Can you work these out from the drawing? Everything is in mm from the part's minimum corner. A direction names the side the tool comes from. Round coordinates to 2 decimals unless told otherwise and drop trailing zeros. Order: outer loops, then holes, each group sorted by start corner. A loop starts at its lowest first (then second) coordinate and runs counter-clockwise, first axis right, second up. Notation, with made-up numbers: M -6.5,14.25 L 36.5,14.25 A15 cw 36.5,40.25 Z; hole C 75,-11 d2. An arc over 180 degrees is marked long. Write each question's results on one line, items separated by ' | '. Start each with the question number.
1. I'm going to push flat-ended pins straight in: pin 1 (1 mm diameter, centred on y = 51.5, z = 5.5, fed in from -X); pin 2 (2 mm diameter, centred on x = 30.5, z = 12.5, fed in from +Y); pin 3 (10 mm diameter, centred on x = 60.5, y = 16, fed in from +Z). Where does each tip first touch, or does it pass through?
2. Suppose I cut it at A-A on x = 10. Write out the boundary of the cut face in (y, z).
3. Suppose I cut it at B-B on y = 68. Write out the boundary of the cut face in (x, z).
4. Suppose I cut it at C-C on z = 9. Write out the boundary of the cut face in (x, y).
5. Please list where these lines run through material, in increasing order: L1, parallel to Z at x = 76, y = 68; L2, parallel to X at y = 34.5, z = 16; L3, parallel to Y at x = 52, z = 14.
6. For the marked faces 1 and 2, which set-ups out of +Z, -Z, +X, -X, +Y, -Y let a thin tool reach every point of the face, with its end or its side?
7. Suppose I cut it at D-D on z = 2.75. Write out the boundary of the cut face in (x, y).
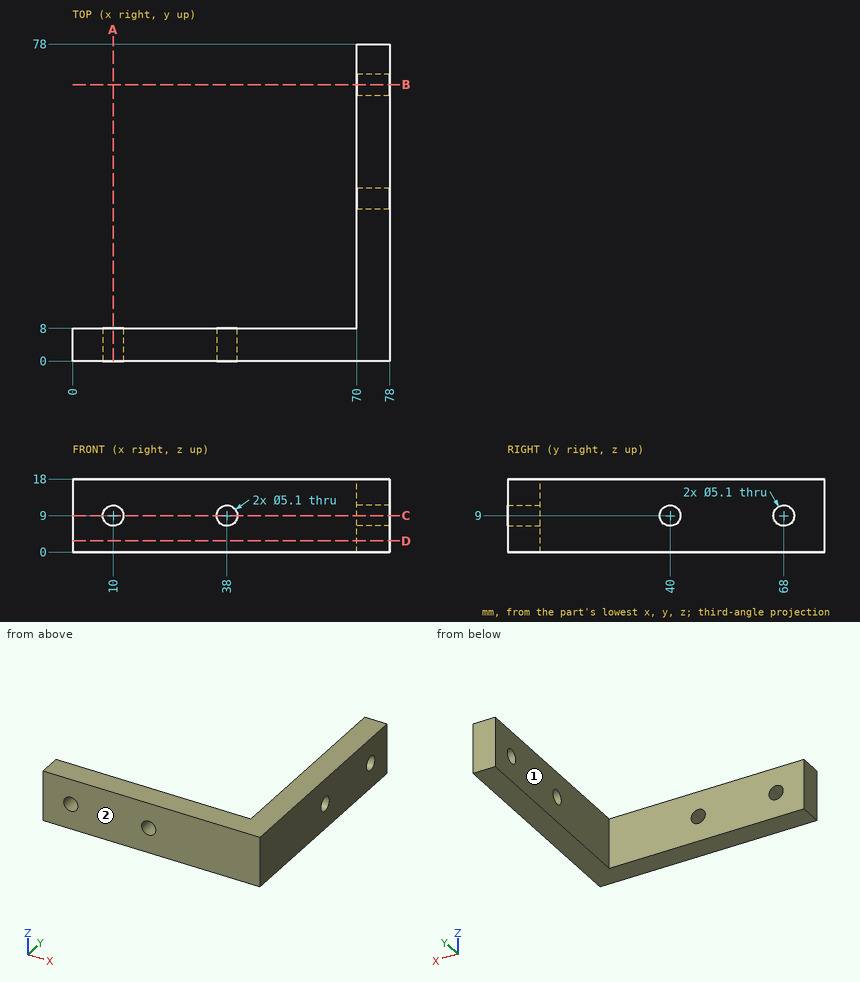
Filled sheet:
1) pin 1: stops at x = 70 | pin 2: stops at y = 8 | pin 3: passes through
2) outline: M 0,0 L 8,0 L 8,6.45 L 0,6.45 Z; M 0,11.55 L 8,11.55 L 8,18 L 0,18 Z
3) outline: M 70,0 L 78,0 L 78,6.45 L 70,6.45 Z; M 70,11.55 L 78,11.55 L 78,18 L 70,18 Z
4) outline: M 0,0 L 7.45,0 L 7.45,8 L 0,8 Z; M 12.55,0 L 35.45,0 L 35.45,8 L 12.55,8 Z; M 40.55,0 L 78,0 L 78,37.45 L 70,37.45 L 70,8 L 40.55,8 Z; M 70,42.55 L 78,42.55 L 78,65.45 L 70,65.45 Z; M 70,70.55 L 78,70.55 L 78,78 L 70,78 Z
5) L1: z = 0 to 6.45, 11.55 to 18 | L2: x = 70 to 78 | L3: y = 0 to 8
6) face 1: +Z, -Z, -X, +Y | face 2: +Z, -Z, +X, -X, -Y
7) outline: M 0,0 L 78,0 L 78,78 L 70,78 L 70,8 L 0,8 Z
